Verification items for this drawing (mm, ordinates from the low corner). Round coordinates to 2 decimals unless told otherwise and drop trailing zeros. Order: outer loops, then holes, each group sorted by start corner. A loop starts at its lowest first (then second) coordinate and runs counter-clockwise, first axis right, second up. Notation, with made-up numbers: M -33,43 L -24,43 A23 cw -24,64 Z; hole C 19,-37.75 d4. An arc over 180 degrees is marked long. One line per item, written item: value. Start each with the question number.
(1) Cross-section at A-A, the plane x = 62. Enter the section's corners in (y, z), and give its area (3 significant figures).
(2) Thickness scan on L1, parallel to Y at x = 117, z = 2.8; L2, parallel to Y at x = 32, z = 2.8; L3, parallel to X at y = 36, z = 2.7. Record the ranges inside material, lowest first.
(3) Cross-section at C-C, the plane y = 12. Enter the section's corners in (x, z), and give its area (3 significant figures).
(4) Cross-section at B-B, the plane z = 1.4. Count the separate pieces of the cut face and the enclosed holes in it, and give its area (3 significant figures).
(5) Cross-section at D-D, the plane y = 31.5. Enter the section's corners in (x, z).
(6) Depth check by flat-ended pin: pin 1 Ø6.5 at (x, y) = (117, 7) entering from -Z; pin 2 Ø6.5 at (x, y) = (32, 12) entering from +Z. Enter the tip coordinate at first touch or a pass-through.
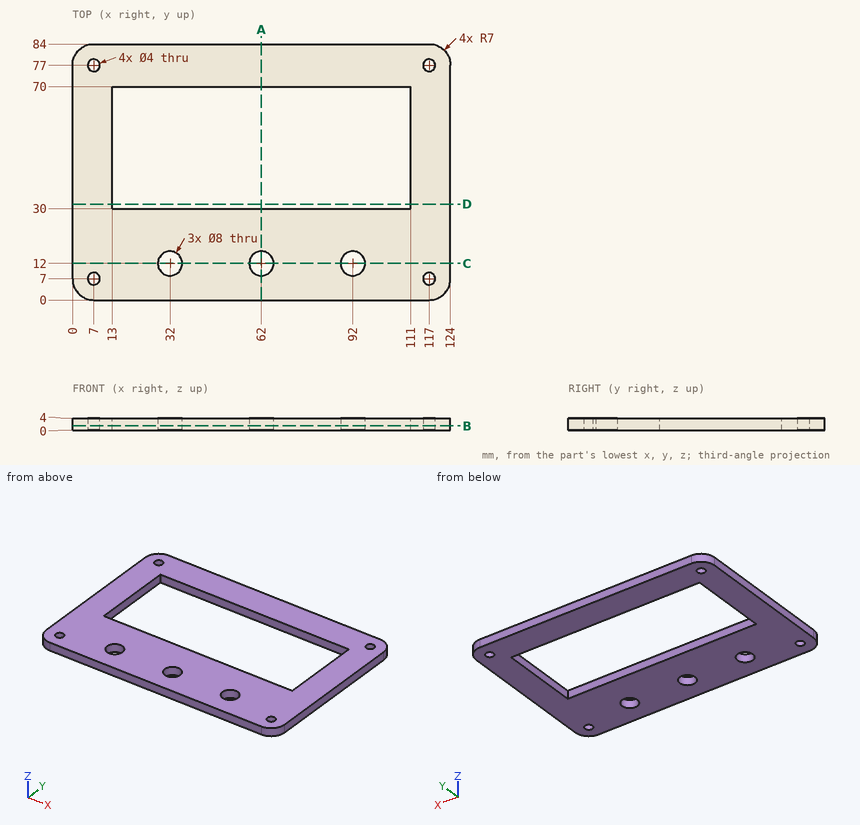
Values found:
1. outline: M 0,0 L 8,0 L 8,4 L 0,4 Z; M 16,0 L 30,0 L 30,4 L 16,4 Z; M 70,0 L 84,0 L 84,4 L 70,4 Z
1. area: 144 mm^2
2. L1: 0 to 5, 9 to 75, 79 to 84
2. L2: 0 to 8, 16 to 30, 70 to 84
2. L3: 0 to 13, 111 to 124
3. outline: M 0,0 L 28,0 L 28,4 L 0,4 Z; M 36,0 L 58,0 L 58,4 L 36,4 Z; M 66,0 L 88,0 L 88,4 L 66,4 Z; M 96,0 L 124,0 L 124,4 L 96,4 Z
3. area: 400 mm^2
4. separate pieces: 1
4. enclosed holes: 8
4. area: 6,250 mm^2
5. outline: M 0,0 L 13,0 L 13,4 L 0,4 Z; M 111,0 L 124,0 L 124,4 L 111,4 Z
6. pin 1: z = 0
6. pin 2: through
